```python
from build123d import *

# Parameters (mm, degrees)
BOSS_EXTRUDE1_DEPTH = 12.7
EXTRUDE_THIN1_START = -6.35
EXTRUDE_THIN1_DEPTH = 12.7
BOSS_EXTRUDE2_DEPTH = 12.7
FILLET2_R           = 20
CHAMFER1_SIZE       = 10


# Read off the part's stored shape, not the designer's step: Extrude-Thin1
with BuildPart() as part:
    # Sketch1 → Boss-Extrude1 (new body)
    with BuildSketch(Plane(origin=(0, 0, 0), x_dir=(0, 0, -1), z_dir=(1, 0, 0))):
        Polygon((72.847962895, 3.175), (72.847962895, 0), (98.247962895, 0), (98.247962895, 38.1), (91.897962895, 38.1), (91.897962895, 6.35), (79.197962895, 6.35), (79.197962895, 38.1), (72.847962895, 38.1), align=None)
    extrude(amount=BOSS_EXTRUDE1_DEPTH)



with BuildPart() as body_2:
    # Extrude-Thin1 outline → Extrude-Thin1 (new body)
    with BuildSketch(Plane(origin=(6.35, 0, 0), x_dir=(0, 0, -1), z_dir=(1, 0, 0)).offset(EXTRUDE_THIN1_START)):
        with BuildLine():
            Line((72.417611424, 0.000950446), (72.262248261, 6.349049554))
            add(Edge.make_bspline(
                [(72.262248261, 6.349049554), (63.021883212, 6.122901173), (54.028914036, 6.667445615), (36.522694485, 9.291097632), (28.009187017, 11.370086401), (11.442378767, 17.064926737), (3.388803369, 20.680920683), (-12.273002956, 29.461644656), (-19.881272632, 34.626626552), (-27.26926203, 40.573319228)],
                knots=[0, 0, 0, 0, 0.25, 0.25, 0.5, 0.5, 0.75, 0.75, 1, 1, 1, 1], degree=3))
            Line((-27.26926203, 40.573319228), (-31.250878284, 35.626680772))
            add(Edge.make_bspline(
                [(72.417611424, 0.000950446), (62.82712633, -0.233766762), (53.463624565, 0.331247938), (35.205660639, 3.067563666), (26.31145557, 5.238983498), (9.011597154, 11.185809829), (0.606218421, 14.961073948), (-15.70112511, 24.103715563), (-23.603051159, 29.470841193), (-31.250878284, 35.626680772)],
                knots=[0, 0, 0, 0, 0.25, 0.25, 0.5, 0.5, 0.75, 0.75, 1, 1, 1, 1], degree=3))
        make_face()
    extrude(amount=EXTRUDE_THIN1_DEPTH)


with BuildPart() as part_1:
    add(part.part)

    add(body_2.part)  # Boss-Extrude2 merges body 2
    # Sketch3 → Boss-Extrude2 (add)
    with BuildSketch(Plane(origin=(12.7, 0, 0), x_dir=(0, 0, -1), z_dir=(1, 0, 0))):
        Polygon((72.262248261, 6.349049554), (72.847962895, 6.349049554), (72.847962895, 0), (72.417611424, 0.000950446), align=None)
    extrude(amount=-BOSS_EXTRUDE2_DEPTH)

    # Fillet2
    fillet2_edges = [part_1.edges().sort_by_distance(p)[0] for p in [
        (6.35, 6.349049554, -72.847962895),
    ]]
    fillet(fillet2_edges, radius=FILLET2_R)

    # Chamfer1
    # the kernel refuses this chamfer: 10 mm, written as the material it adds along each edge
    with BuildSketch(Plane(origin=(0, 6.35, -91.897962895), x_dir=(0, -0.027495876610586664, 0.9996219169112968), z_dir=(1, 0, 0)), Plane(origin=(0, 6.35, -79.197962895), x_dir=(0, 0.9996219169112968, 0.027495876610586317), z_dir=(1, 0, 0))) as chamfer1_piece_1:
        Polygon((CHAMFER1_SIZE * 0.999621916911, -CHAMFER1_SIZE * 0.0274958766106), (-CHAMFER1_SIZE * 0.0274958766106, -CHAMFER1_SIZE * 0.999621916911), (0, 0), align=None)
    extrude(amount=12.7)


solid = part_1.part
```
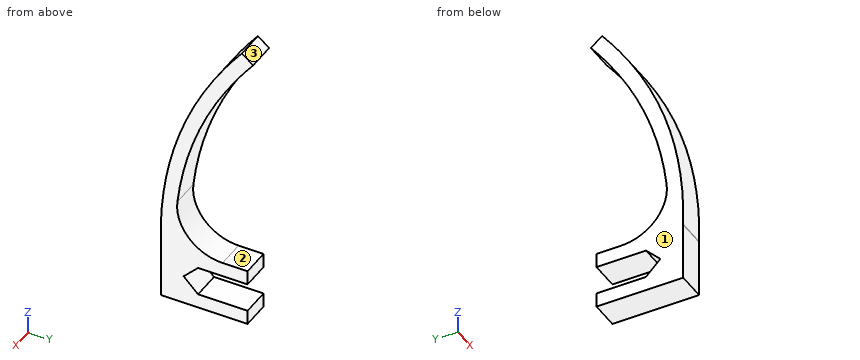
Input: part model. Units: mm. Frame: model coordinates. Face numbers are marked on the shaded views. Give positions to 0.01 mm unless a question says otherwise; leave off trailing zeros. Order: outer loops, then holes, each group sorted by start corner. A loop starts at its lowest first (then second) coordinate and runs counter-clockwise, first axis right, second up. Notation, with made-up numbers: (78, 54.5) - (87, 54.5) arc R19 ccw to (87, 59.5) - close; hole circle Ø3 at (64.5, 59.25). An arc over 180 degrees is marked (long way). Use a Markdown table: item, result.
(1) Draft query along Z for the marked faces 1, 2 and 3. Return one class per face: released by +Z, released by -Z, zero draft, split by the parting line, or undercut.
Computed values:
| item | result |
|---|---|
| face 1 | zero draft |
| face 2 | undercut |
| face 3 | released by +Z |
(2) Section query A-A (y = 30.5). State how many separate pieces and enclosed holes the cut face has, then the cut area to 3 significant figures.
Computed values:
| item | result |
|---|---|
| separate pieces | 3 |
| enclosed holes | 0 |
| area | 303 mm2 |
(3) Pin query (flat end, axial travel): pin 1 (1.5 mm diameter, centred on x = 3, z = -40.5, fed in from -Y); pin 2 (5 mm diameter, centred on x = 9.5, z = -94, fed in from +Y); pin 3 (4 mm diameter, centred on x = 11, z = -12, fed in from +Y). Return the tip coordinate at first contact, or that it passes through.
Computed values:
| item | result |
|---|---|
| pin 1 | stops at y = 2.19 |
| pin 2 | stops at y = 38.1 |
| pin 3 | stops at y = 17.96 |
(4) Section query B-B (z = -82.5). Output: boundary loops of the cut face in (x, y).
Computed values:
| item | result |
|---|---|
| outline | (0, 0) - (12.7, 0) - (12.7, 13.05) - (0, 13.05) - close |
(5) Line query: line 1 (Z direction, x = 11, y = 22.5); line 2 (Z direction, x = 1, y = 36); line 3 (Y direction, x = 3.5, z = -76). Output: solid intervals per line, ascending. Write a range as from..to.
Computed values:
| item | result |
|---|---|
| line 1 | z = -98.25..-91.9, -79.2..-72.3, -0.34..12.62 |
| line 2 | z = -98.25..-91.9, -79.2..-72.85, 21.34..30.95 |
| line 3 | y = 0..38.1 |
